Job drawing, mm, ordinate dimensions from the low corner. One solid piece. Round coordinates to 2 decimals unless told otherwise and drop trailing zeros. Loops run counter-clockwise (first coordinate to the right, second up) from the corner with the lowest first, then second, coordinate; pieces in that order, holes last. Notation, with made-up numbers: (-13.5, -7) - (1.5, -7) arc R28 ccw to (1.5, 19) - close; hole circle Ø5 at (60.25, 22). An arc over 180 degrees is marked (long way). One line per question, with ' | ' between items. Start each with the question number.
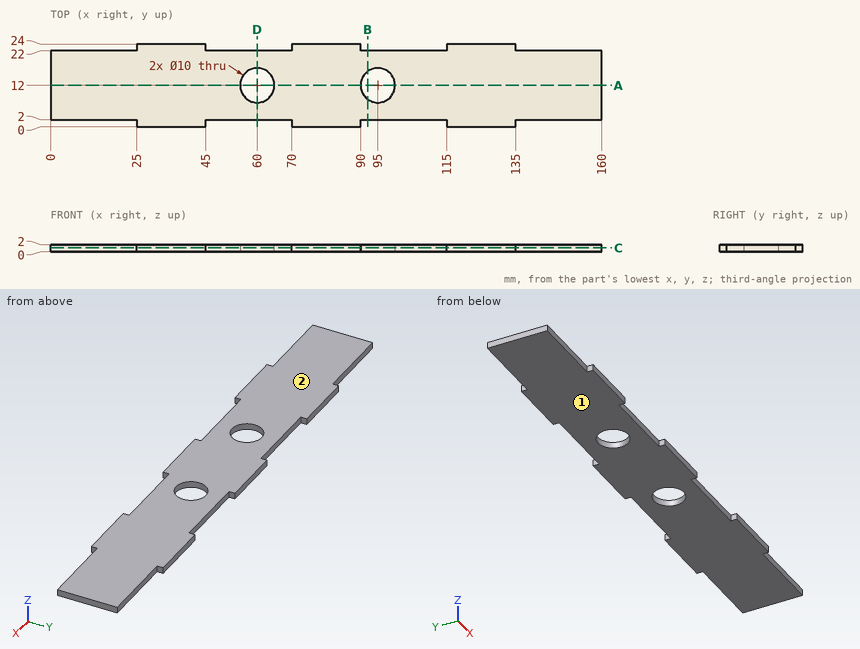
1) Two-plate mould, pull along Z, no slides. Class the marked faces 1 and 2: +Z half, -Z half, draft (parallel to the pull), parting line (faces both ways), or undercut.
2) Wall check: line 1 (X direction, y = 1, z = 1.3); line 2 (Y direction, x = 95, z = 1); line 3 (X direction, y = 10, z = 1.05). Give the ranges that are in metal, low to high. Write a range as [from, to].
3) Saw through at D-D on x = 60. Write the cut outline in (y, z).
4) Drop flat-ended pins along their axis: pin 1 (0.6 mm diameter, centred on y = 23, z = 0.5, fed in from -X); pin 2 (0.6 mm diameter, centred on x = 103, z = 0.5, fed in from +Y); pin 3 (8 mm diameter, centred on x = 95, y = 12, fed in from +Z). Give the stop position or say it passes through.
5) Saw through at C-C on z = 1.1. State how many separate pieces and enclosed holes the cut face has, and give its area (3 significant figures).
6) Saw through at A-A on y = 12. Write the cut outline in (x, z), and give its area (3 significant figures).
7) Saw through at B-B on x = 92. Write the cut outline in (y, z), and give its area (3 significant figures).
Answer key:
1) face 1: -Z half | face 2: +Z half
2) line 1: [25, 45], [70, 90], [115, 135] | line 2: [2, 7], [17, 22] | line 3: [0, 55.42], [64.58, 90.42], [99.58, 160]
3) outline: (2, 0) - (7, 0) - (7, 2) - (2, 2) - close; (17, 0) - (22, 0) - (22, 2) - (17, 2) - close
4) pin 1: x = 25 | pin 2: y = 22 | pin 3: through
5) separate pieces: 1 | enclosed holes: 2 | area: 3,280 mm²
6) outline: (0, 0) - (55, 0) - (55, 2) - (0, 2) - close; (65, 0) - (90, 0) - (90, 2) - (65, 2) - close; (100, 0) - (160, 0) - (160, 2) - (100, 2) - close | area: 280 mm²
7) outline: (2, 0) - (8, 0) - (8, 2) - (2, 2) - close; (16, 0) - (22, 0) - (22, 2) - (16, 2) - close | area: 24.0 mm²
